```python
from build123d import *

# Parameters (mm, degrees)
SKIZZE1_R                       = 12
SKIZZE1_R_2                     = 1.7
AUFSATZ_LINEAR_AUSTRAGEN1_DEPTH = 17
SKIZZE3_R                       = 3.5
SCHNITT_LINEAR_AUSTRAGEN1_DEPTH = 12


with BuildPart() as part:
    # Skizze1 → Aufsatz-Linear austragen1 (new body)
    with BuildSketch(Plane.XY):
        Circle(SKIZZE1_R)
        with Locations((5.656854249, 5.656854249)):
            Circle(SKIZZE1_R_2, mode=Mode.SUBTRACT)
        with Locations((-5.656854249, 5.656854249)):
            Circle(SKIZZE1_R_2, mode=Mode.SUBTRACT)
        with Locations((-5.656854249, -5.656854249)):
            Circle(SKIZZE1_R_2, mode=Mode.SUBTRACT)
        with Locations((5.656854249, -5.656854249)):
            Circle(SKIZZE1_R_2, mode=Mode.SUBTRACT)
        with BuildLine():
            ThreePointArc((3.815756806, -1.5), (-4.1, 0), (3.815756806, 1.5))
            Line((3.815756806, 1.5), (5.3, 1.5))
            Line((5.3, 1.5), (5.3, -1.5))
            Line((5.3, -1.5), (3.815756806, -1.5))
        make_face(mode=Mode.SUBTRACT)
    extrude(amount=AUFSATZ_LINEAR_AUSTRAGEN1_DEPTH)

    # Skizze3 → Schnitt-Linear austragen1 (cut)
    with BuildSketch(Plane(origin=(0, 0, 0), x_dir=(-1, 0, 0), z_dir=(0, 0, -1))):
        with Locations((-5.656854249, 5.656854249)):
            Circle(SKIZZE3_R)
        with Locations((5.656854249, 5.656854249)):
            Circle(SKIZZE3_R)
        with Locations((5.656854249, -5.656854249)):
            Circle(SKIZZE3_R)
        with Locations((-5.656854249, -5.656854249)):
            Circle(SKIZZE3_R)
    extrude(amount=-SCHNITT_LINEAR_AUSTRAGEN1_DEPTH, mode=Mode.SUBTRACT)


solid = part.part
```
Input: part model. Units: mm. Frame: model coordinates. A direction names the side the tool comes from. Coordinates: 2 decimals unless noted, no trailing zeros. Write each loop counter-clockwise with the first axis right and the second up, starting at its lowest first coordinate (ties: lowest second). Pieces come first, ordered by that corner, then holes. Notation, with made-up numbers: M 49.5,73 L 62.5,73 A21 ccw 62.5,80 Z; hole C 18.5,68.25 d2. An arc over 180 degrees is marked long. Use one line per item in the form item = value.
Q1. Section B-B (x = 0.25). Return loops of the section in (y, z), plus the area to 3 significant figures.
Answer below:
outline = M -12,0 L -4.09,0 L -4.09,17 L -12,17 Z; M 4.09,0 L 12,0 L 12,17 L 4.09,17 Z
area = 269 mm²
Q2. Material intervals for probe 1 along X at (y, z) = (-8.75, 7.75); probe 2 along X at (y, z) = (7.5, 5.5); probe 3 along Y at (x, z) = (0, 7.5), sorted ascending. Write a range as from..to.
Answer below:
probe_1 = -8.21..-7.29, -4.02..4.02, 7.29..8.21
probe_2 = -9.37..-8.63, -2.68..2.68, 8.63..9.37
probe_3 = -12..-4.1, 4.1..12
Q3. Section A-A (y = 0). Return loops of the section in (x, z), plus the area to 3 significant figures.
Answer below:
outline = M -12,0 L -4.1,0 L -4.1,17 L -12,17 Z; M 5.3,0 L 12,0 L 12,17 L 5.3,17 Z
area = 248 mm²
Q4. First-contact query: pin 1 (2 mm diameter, centred on x = -5, y = -5, fed in from -Z); pin 2 (2 mm diameter, centred on x = 5.66, y = 5.66, fed in from -Z); pin 3 (1.2 mm diameter, centred on x = 4, z = 12, fed in from +Y); pin 4 (10 mm diameter, centred on x = -6, z = 13, fed in from +Y). Flat tips, straight axial feed; report the tip coordinate or a pass-through.
Answer below:
pin_1 = 12
pin_2 = through
pin_3 = 11.51
pin_4 = 11.96
Q5. Set-up query: faces 1 (the face through (-4.898, -9.074, 5.916)), 2 (the face through (5.3, 0, 8)), 3 (the face through (0, -5, 0)). Return all of +Z, -Z, +X, -X, +Y, -Y with unobstructed straight access to the full face (end or side cutting, diameter ignored); none if empty.
Answer below:
face_1 = -Z
face_2 = +Z, -Z
face_3 = -Z, +X, -X, +Y, -Y
Q6. Section D-D (x = -7). Return loops of the section in (y, z).
Answer below:
outline = M -9.75,0 L -8.89,0 L -8.89,12 L -6.7,12 L -6.7,17 L -9.75,17 Z; M -4.61,12 L -2.42,12 L -2.42,0 L 2.42,0 L 2.42,12 L 4.61,12 L 4.61,17 L -4.61,17 Z; M 6.7,12 L 8.89,12 L 8.89,0 L 9.75,0 L 9.75,17 L 6.7,17 Z
Q7. Section C-C (z = 7). Return loops of the section in (x, y), plus the area to 3 significant figures.
Answer below:
outline = C 0,0 d24; hole C -5.66,-5.66 d7; hole C -5.66,5.66 d7; hole C 5.66,-5.66 d7; hole C 5.66,5.66 d7; hole M 3.82,-1.5 L 5.3,-1.5 L 5.3,1.5 L 3.82,1.5 A4.1 ccw long Z
area = 242 mm²
Q8. Draft query along X for faces 4 (the face through (-11.99, 0.53, 8.38)), 5 (the face through (-2.16, 5.81, 5.92)), 6 (the face through (0, -5, 17)), 7 (the face through (5, 1.5, 8)). Return one class per face: released by +X, released by -X, zero draft, split by the parting line, or undercut.
Answer below:
face_4 = split by the parting line
face_5 = undercut
face_6 = zero draft
face_7 = undercut
